```python
from build123d import *

# Parameters (mm, degrees)
Y_KSEKLIK_EKSTR_ZYON1_DEPTH = 220
IZIM2_W                     = 840
IZIM2_H                     = 650
Y_KSEKLIK_EKSTR_ZYON2_DEPTH = 460
KES_EKSTR_ZYON1_DEPTH       = 270
RADYUS2_R                   = 150
RADYUS3_R                   = 150


with BuildPart() as part:
    # Çizim1 → Yükseklik-Ekstrüzyon1 (new body)
    with BuildSketch(Plane.XY):
        with BuildLine():
            Line((-640, 460), (640, 460))
            ThreePointArc((640, 460), (710.710678119, 430.710678119), (740, 360))
            Line((740, 360), (740, 100))
            ThreePointArc((740, 100), (710.710678119, 29.289321881), (640, 0))
            Line((640, 0), (-640, 0))
            ThreePointArc((-640, 0), (-710.710678119, 29.289321881), (-740, 100))
            Line((-740, 100), (-740, 360))
            ThreePointArc((-740, 360), (-710.710678119, 430.710678119), (-640, 460))
        make_face()
    extrude(amount=Y_KSEKLIK_EKSTR_ZYON1_DEPTH)

    # Çizim2 → Yükseklik-Ekstrüzyon2 (add)
    with BuildSketch(Plane(origin=(0, 460, 0), x_dir=(1, 0, 0), z_dir=(0, 1, 0))):
        with Locations((0, 325)):
            Rectangle(IZIM2_W, IZIM2_H)
    extrude(amount=-Y_KSEKLIK_EKSTR_ZYON2_DEPTH)

    # Çizim3 → Kes-Ekstrüzyon1 (cut)
    with BuildSketch(Plane(origin=(0, 460, 0), x_dir=(1, 0, 0), z_dir=(0, 1, 0))):
        with BuildLine():
            Line((0, 70), (0, 650))
            Line((0, 650), (-230, 650))
            Line((-230, 650), (-230, 150))
            ThreePointArc((-230, 150), (-206.568542495, 93.431457505), (-150, 70))
            Line((-150, 70), (0, 70))
        make_face()
        with BuildLine():
            Line((230, 650), (0, 650))
            Line((0, 650), (0, 70))
            Line((0, 70), (150, 70))
            ThreePointArc((150, 70), (206.568542495, 93.431457505), (230, 150))
            Line((230, 150), (230, 650))
        make_face()
    extrude(amount=-KES_EKSTR_ZYON1_DEPTH, mode=Mode.SUBTRACT)

    # Radyus2
    radyus2_edges = [part.edges().sort_by_distance(p)[0] for p in [
        (-325, 460, -650),
    ]]
    fillet(radyus2_edges, radius=RADYUS2_R)

    # Radyus3
    radyus3_edges = [part.edges().sort_by_distance(p)[0] for p in [
        (325, 460, -650),
    ]]
    fillet(radyus3_edges, radius=RADYUS3_R)


solid = part.part
```
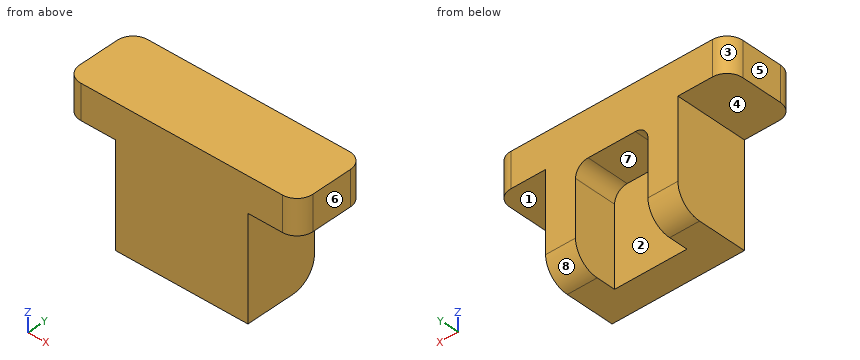
Input: part model. Units: mm. Frame: model coordinates. Face numbers are marked on the shaded views. A direction names the side the tool comes from. Coordinates: 2 decimals unless noted, no trailing zeros. Write each loop counter-clockwise with the first axis right and the second up, starting at its lowest first coordinate (ties: lowest second). Pieces come first, ordered by that corner, then holes. Notation, with made-up numbers: M 57,-7 L 75,-7 A35 cw 75,30 Z; hole C 75,-1.75 d10. An arc over 180 degrees is marked long. Use one line per item in the form item = value.
Q1. Material intervals for probe 1 along X at (y, z) = (230, -251.5); probe 2 along X at (y, z) = (100.5, -120.5); probe 3 along Z at (x, y) = (74, 260.5), sorted ascending. Write a range as from..to.
Answer below:
probe_1 = -420..-230, 230..420
probe_2 = -420..420
probe_3 = -70..220
Q2. Section B-B (z = -382). Return loops of the section in (x, y), plus the area to 3 significant figures.
Answer below:
outline = M -420,0 L 420,0 L 420,460 L 230,460 L 230,190 L -230,190 L -230,460 L -420,460 Z
area = 262,000 mm²
Q3. Draft query along X for the marked faces 6, 7 and 8. Return one class per face: released by +X, released by -X, zero draft, split by the parting line, or undercut.
Answer below:
face_6 = released by +X
face_7 = undercut
face_8 = zero draft
Q4. First-contact query: pin 1 (12 mm diameter, centred on x = -135, z = -483, fed in from +Y); pin 2 (1.5 mm diameter, centred on y = 224.5, z = -277, fed in from +X). Flat tips, straight axial feed; report the tip coordinate or a pass-through.
Answer below:
pin_1 = 190
pin_2 = 420
Q5. Section D-D (y = 133). Return loops of the section in (x, z), plus the area to 3 significant figures.
Answer below:
outline = M -740,0 L -420,0 L -420,-650 L 420,-650 L 420,0 L 740,0 L 740,220 L -740,220 Z
area = 872,000 mm²
Q6. Section C-C (x = -207). Return loops of the section in (y, z).
Answer below:
outline = M 0,-650 L 190,-650 L 190,-93.87 L 460,-93.87 L 460,220 L 0,220 Z
Q7. Set-up query: the marked faces 1, 2, 3, 4 and 5. Return all of +Z, -Z, +X, -X, +Y, -Y with unobstructed straight access to the full face (end or side cutting, diameter ignored); none if empty.
Answer below:
face_1 = -Z, +X, +Y, -Y
face_2 = -Z, +Y
face_3 = +Z, -Z, -X, +Y
face_4 = -Z, -X, +Y, -Y
face_5 = +Z, -Z, -X, +Y, -Y
Q8. Section A-A (y = 288.5). Return loops of the section in (x, z), plus the area to 3 significant figures.
Answer below:
outline = M -740,0 L -420,0 L -420,-650 L -230,-650 L -230,-150 A80 cw -150,-70 L 150,-70 A80 cw 230,-150 L 230,-650 L 420,-650 L 420,0 L 740,0 L 740,220 L -740,220 Z
area = 608,000 mm²
